Here's how the part is built. I have some questions about the finished solid (model axes, mm). Coordinates: 2 decimals unless noted, no trailing zeros. Order: outer loops, then holes, each group sorted by start corner. A loop starts at its lowest first (then second) coordinate and runs counter-clockwise, first axis right, second up. Notation, with made-up numbers: (11.25, -27.75) - (40.25, -27.75) arc R33 cw to (40.25, 6.25) - close; hole circle Ø10 at (-21, 87.5). An arc over 180 degrees is marked (long way). Use one line per item in the form item = value. Start each with the question number.
Autodesk Fusion 360 part; units mm, degrees
sketch "Sketch1" plane through (0, 0, 0) normal (0, 0, 1) x (1, 0, 0)
  line L0 (3.7286, -31.8797) -> (3.7286, -35.8797)
  line L1 (3.7286, -35.8797) -> (-16.2714, -35.8797)
  line L2 (-16.2714, -35.8797) -> (-16.2714, -31.8797)
  line L3 (54.8886, -31.8797) -> (54.8886, -35.8797)
  line L4 (54.8886, -35.8797) -> (34.8886, -35.8797)
  line L5 (34.8886, -35.8797) -> (34.8886, -31.8797)
  line L6 (110.3886, -31.8797) -> (110.3886, -35.8797)
  line L7 (110.3886, -35.8797) -> (90.3886, -35.8797)
  line L8 (90.3886, -35.8797) -> (90.3886, -31.8797)
  line L9 (159.5486, -31.8797) -> (159.5486, -35.8797)
  line L10 (159.5486, -35.8797) -> (139.5486, -35.8797)
  line L11 (139.5486, -35.8797) -> (139.5486, -31.8797)
  line L12 (190.7086, -31.8797) -> (190.7086, -35.8797)
  line L13 (190.7086, -35.8797) -> (210.7086, -35.8797)
  line L14 (210.7086, -35.8797) -> (210.7086, -31.8797)
  line L15 (239.5686, -31.8797) -> (235.3824, -31.8797)
  line L16 (235.3824, -31.8797) -> (210.7086, -31.8797)
  line L17 (190.7086, -31.8797) -> (187.1012, -31.8797)
  line L18 (187.1012, -31.8797) -> (159.5486, -31.8797)
  line L19 (139.5486, -31.8797) -> (110.3886, -31.8797)
  line L20 (90.3886, -31.8797) -> (54.8886, -31.8797)
  line L21 (34.8886, -31.8797) -> (29.9892, -31.8797)
  line L22 (29.9892, -31.8797) -> (3.7286, -31.8797)
  line L23 (-16.2714, -31.8797) -> (-45.4314, -31.8797)
  line L24 (159.5686, 48.1203) -> (159.5686, 33.1203)
  line L25 (159.5686, 33.1203) -> (219.5686, 33.1203)
  line L26 (219.5686, 33.1203) -> (219.5686, 48.1203)
  line L27 (34.5686, 48.1203) -> (34.5686, 33.1203)
  line L28 (34.5686, 33.1203) -> (-25.4314, 33.1203)
  line L29 (-25.4314, 33.1203) -> (-25.4314, 48.1203)
  line L30 (239.5686, 48.1203) -> (219.5686, 48.1203)
  line L31 (159.5686, 48.1203) -> (34.5686, 48.1203)
  line L32 (-25.4314, 48.1203) -> (-45.4314, 48.1203)
  line L33 (-45.4314, -6.8797) -> (-41.4314, -6.8797)
  line L34 (-41.4314, -6.8797) -> (-41.4314, 23.1203)
  line L35 (-41.4314, 23.1203) -> (-45.4314, 23.1203)
  line L36 (-45.4314, -31.8797) -> (-45.4314, -27.5346)
  line L37 (-45.4314, -27.5346) -> (-45.4314, -6.8797)
  line L38 (-45.4314, 23.1203) -> (-45.4314, 26.6822)
  line L39 (-45.4314, 26.6822) -> (-45.4314, 48.1203)
  line L40 (-45.4314, -6.8797) -> (-41.4314, -6.8797)
  line L41 (-41.4314, -6.8797) -> (-41.4314, 23.1203)
  line L42 (-45.4314, 23.1203) -> (-45.4314, 26.6822)
  line L43 (-41.4314, 23.1203) -> (-45.4314, 23.1203)
  line L44 (239.5686, 23.1203) -> (235.5686, 23.1203)
  line L45 (235.5686, -6.8797) -> (239.5686, -6.8797)
  line L46 (239.5686, 23.1203) -> (235.5686, 23.1203)
  line L47 (235.5686, -6.8797) -> (239.5686, -6.8797)
  line L48 (235.5686, 23.1203) -> (235.5686, -6.8797)
  line L49 (239.5686, 23.1203) -> (239.5686, 48.1203)
  line L50 (239.5686, -31.8797) -> (239.5686, -30.1367)
  line L51 (239.5686, -30.1367) -> (239.5686, -6.8797)
  line L52 (-8.2714, -6.8797) -> (-4.2714, -6.8797)
  line L53 (-4.2714, -6.8797) -> (-4.2714, 23.1203)
  line L54 (-4.2714, 23.1203) -> (-8.2714, 23.1203)
  line L55 (-8.2714, 23.1203) -> (-8.2714, -6.8797)
  line L56 (42.8886, -6.8797) -> (46.8886, -6.8797)
  line L57 (46.8886, -6.8797) -> (46.8886, 23.1203)
  line L58 (46.8886, 23.1203) -> (42.8886, 23.1203)
  line L59 (42.8886, 23.1203) -> (42.8886, -6.8797)
  line L60 (98.0886, -6.8797) -> (102.0886, -6.8797)
  line L61 (102.0886, -6.8797) -> (102.0886, 23.1203)
  line L62 (102.0886, 23.1203) -> (98.0886, 23.1203)
  line L63 (98.0886, 23.1203) -> (98.0886, -6.8797)
  line L64 (147.2486, -6.8797) -> (151.2486, -6.8797)
  line L65 (151.2486, -6.8797) -> (151.2486, 23.1203)
  line L66 (151.2486, 23.1203) -> (147.2486, 23.1203)
  line L67 (147.2486, 23.1203) -> (147.2486, -6.8797)
  line L68 (198.4086, -6.8797) -> (202.4086, -6.8797)
  line L69 (202.4086, -6.8797) -> (202.4086, 23.1203)
  line L70 (202.4086, 23.1203) -> (198.4086, 23.1203)
  line L71 (198.4086, 23.1203) -> (198.4086, -6.8797)
extrude "Extrude1" add sketch "Sketch1" along normal blind 4
1) I need wall thicknesses on probe 1 along X at (y, z) = (-4, 2.2); probe 2 along X at (y, z) = (39, 0.8); probe 3 along Y at (x, z) = (129, 0.9). Which ranges of each line are inside material? Lowest first, please. Write a range as [from, to].
2) For pin 1 (2 mm diameter, centred on x = 57.5, z = 2.5, fed in from -Y); pin 2 (2 mm diameter, centred on y = -34.5, z = 1.5, fed in from -X); pin 3 (1.2 mm diameter, centred on y = 2.5, z = 1.5, fed in from +X), each with a flat end and sliding along its axis, tell me the tip position at first contact or that it passes through.
3) Suppose I cut it at C-C, the plane x = 20.5. List the corners of the cut face in (y, z) for me.
4) Suppose I cut it at B-B, the plane z = 2.35. Give the number of separate pieces and of enclosed holes in the cut face, then the cut area to 3 significant figures.
5) Suppose I cut it at D-D, the plane x = 119.5. List the corners of the cut face in (y, z) for me.
6) Suppose I cut it at A-A, the plane y = 13. List the corners of the cut face in (x, z) for me, then the cut area to 3 significant figures.
From the geometry:
q1.probe_1 = [-41.43, -8.27], [-4.27, 42.89], [46.89, 98.09], [102.09, 147.25], [151.25, 198.41], [202.41, 235.57]
q1.probe_2 = [-45.43, -25.43], [34.57, 159.57], [219.57, 239.57]
q1.probe_3 = [-31.88, 48.12]
q2.pin_1 = -31.88
q2.pin_2 = -16.27
q2.pin_3 = 235.57
q3.outline = (-31.88, 0) - (33.12, 0) - (33.12, 4) - (-31.88, 4) - close
q4.separate_pieces = 1
q4.enclosed_holes = 5
q4.area = 20,600 mm2
q5.outline = (-31.88, 0) - (48.12, 0) - (48.12, 4) - (-31.88, 4) - close
q6.outline = (-41.43, 0) - (-8.27, 0) - (-8.27, 4) - (-41.43, 4) - close; (-4.27, 0) - (42.89, 0) - (42.89, 4) - (-4.27, 4) - close; (46.89, 0) - (98.09, 0) - (98.09, 4) - (46.89, 4) - close; (102.09, 0) - (147.25, 0) - (147.25, 4) - (102.09, 4) - close; (151.25, 0) - (198.41, 0) - (198.41, 4) - (151.25, 4) - close; (202.41, 0) - (235.57, 0) - (235.57, 4) - (202.41, 4) - close
q6.area = 1,030 mm2
